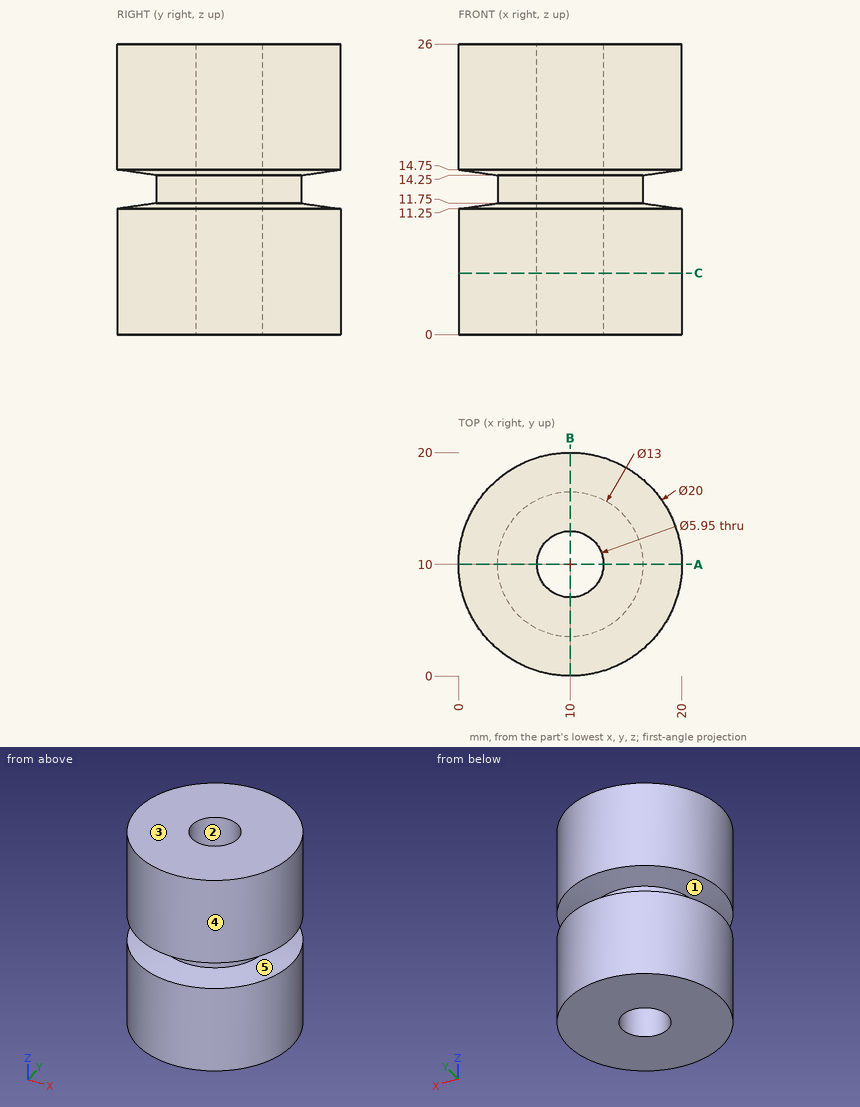
Drawing for the job (mm, zero at the part's lowest x, y, z). A direction names the side the tool comes from. Round coordinates to 2 decimals unless told otherwise and drop trailing zeros. Order: outer loops, then holes, each group sorted by start corner. A loop starts at its lowest first (then second) coordinate and runs counter-clockwise, first axis right, second up. Notation, with made-up numbers: (-5.5, 47) -> (28.5, 47) arc R13 ccw to (28.5, 64) -> close; hole circle Ø10 at (-19, 53). An arc over 180 degrees is marked (long way). Put each result on its own line as item: value.
Q1. Pin check, flat tips, straight feed: pin 1 Ø5 at (x, y) = (10, 10) entering from -Z; pin 2 Ø12 at (y, z) = (16.5, 12.5) entering from +X; pin 3 Ø3 at (x, z) = (18, 17) entering from -Y; pin 4 Ø3 at (x, z) = (5.5, 9.5) entering from -Y. Stop position of each tip, or through.
From the geometry:
pin 1: passes through
pin 2: stops at x = 19.98
pin 3: stops at y = 2.4
pin 4: stops at y = 0.46
Q2. Band-saw the part on A-A (y = 10). Give the cut face in (x, z) (3 decimals), and give its area (3 significant figures).
From the geometry:
outline: (0, 0) -> (7.025, 0) -> (7.025, 26) -> (0, 26) -> (0, 14.75) -> (3.5, 14.25) -> (3.5, 11.75) -> (0, 11.25) -> close; (12.975, 0) -> (20, 0) -> (20, 11.25) -> (16.5, 11.75) -> (16.5, 14.25) -> (20, 14.75) -> (20, 26) -> (12.975, 26) -> close
area: 344 mm2
Q3. Wall check: line 1 (Y direction, x = 10, z = 9.75) (3 decimals); line 2 (Z direction, x = 1.5, y = 12.5); line 3 (Z direction, x = 3.75, y = 4.75). Give the ranges that are in metal, low to high. Write a range as [from, to].
From the geometry:
line 1: y = [0, 7.025], [12.975, 20]
line 2: z = [0, 11.41], [14.59, 26]
line 3: z = [0, 11.51], [14.49, 26]
Q4. Pull direction X, two halves, no side cores. Call the marked faces 1, 2 and 3: pulls with the +X half, pulls with the -X half, needs draft (parallel to the pull), parting line crosses it, or undercut.
From the geometry:
face 1: parting line crosses it
face 2: undercut
face 3: needs draft
Q5. Tool access for the marked faces 4 and 5: list every direction of +Z, -Z, +X, -X, +Y, -Y with a clear straight run to the whole face (end or side of a thin tool).
From the geometry:
face 4: +Z, -Z
face 5: none
Q6. Band-saw the part on C-C (z = 5.5). Give the cut face in (x, y) (3 decimals), and give its area (3 significant figures).
From the geometry:
outline: circle Ø20 at (10, 10); hole circle Ø5.95 at (10, 10)
area: 286 mm2
